```python
from build123d import *

# Parameters (mm, degrees)
SKETCH_W        = 110
SKETCH_H        = 25
PAD_DEPTH       = 70
POCKET_DEPTH    = 22.5
SKETCH002_W     = 20
SKETCH002_H     = 22.5
POCKET001_DEPTH = 70.001
SKETCH003_W     = 15
SKETCH003_H     = 15
SKETCH003_R     = 1.5
PAD001_DEPTH    = 2.5
SKETCH004_W     = 15
SKETCH004_H     = 15
SKETCH004_R     = 1.5
PAD002_DEPTH    = 2.5
POCKET002_DEPTH = 2.5
SKETCH006_W     = 26
SKETCH006_H     = 14.5
POCKET003_DEPTH = 2.5
SKETCH007_W     = 20
SKETCH007_H     = 2.5
PAD003_DEPTH    = 22.5
SKETCH008_W     = 20
SKETCH008_H     = 2.5
PAD004_DEPTH    = 22.5
SKETCH009_R     = 1.5
PAD005_DEPTH    = 0.15
SKETCH010_R     = 1.5
PAD006_DEPTH    = 0.15


with BuildPart() as part:
    # Sketch → Pad (new body)
    with BuildSketch(Plane.YZ):
        with Locations((55, 12.5)):
            Rectangle(SKETCH_W, SKETCH_H)
    extrude(amount=PAD_DEPTH)

    # Sketch001 (on Face3 of Pad) → Pocket (cut)
    with BuildSketch(Plane(origin=(0, 0, 25), x_dir=(0, -1, 0), z_dir=(0, 0, 1))):
        Polygon((-107.5, 2.5), (-2.5, 2.5), (-2.5, 67.5), (-107.5, 67.5), (-110, 67.5), (-110, 2.5), align=None)
    extrude(amount=-POCKET_DEPTH, mode=Mode.SUBTRACT)

    # Sketch002 (on Face5 of Pocket) → Pocket001 (cut, through all)
    with BuildSketch(Plane.YZ.offset(70)):
        with Locations((100, 13.75)):
            Rectangle(SKETCH002_W, SKETCH002_H)
    extrude(amount=-POCKET001_DEPTH, mode=Mode.SUBTRACT)

    # Sketch003 (on Face5 of Pocket001) → Pad001 (join, symmetric)
    with BuildSketch(Plane.YZ.offset(70)):
        with Locations((40, 27.5)):
            Rectangle(SKETCH003_W, SKETCH003_H)
        with Locations((40, 30)):
            Circle(SKETCH003_R, mode=Mode.SUBTRACT)
    extrude(amount=PAD001_DEPTH, both=True)

    # Sketch004 (on Face4 of Pad001) → Pad002 (join, symmetric)
    with BuildSketch(Plane(origin=(0, 0, 0), x_dir=(0, 1, 0), z_dir=(-1, 0, 0))):
        with Locations((40, -27.5)):
            Rectangle(SKETCH004_W, SKETCH004_H)
        with Locations((40, -30)):
            Circle(SKETCH004_R, mode=Mode.SUBTRACT)
    extrude(amount=PAD002_DEPTH, both=True)

    # Sketch005 → Pocket002 (cut)
    with BuildSketch(Plane.YX):
        with BuildLine():
            ThreePointArc((70, 47.5), (57.5, 35), (70, 22.5))
            Line((70, 22.5), (110, 22.5))
            ThreePointArc((110, 22.5), (122.5, 35), (110, 47.5))
            Line((70, 47.5), (110, 47.5))
        make_face()
    extrude(amount=-POCKET002_DEPTH, mode=Mode.SUBTRACT)

    # Sketch006 (on Face2 of Pocket002) → Pocket003 (cut)
    with BuildSketch(Plane(origin=(0, 0, 0), x_dir=(0, 1, 0), z_dir=(-1, 0, 0))):
        with Locations((77, -17.75)):
            Rectangle(SKETCH006_W, SKETCH006_H)
    extrude(amount=-POCKET003_DEPTH, mode=Mode.SUBTRACT)

    # Sketch007 (on Face17 of Pocket003) → Pad003 (join)
    with BuildSketch(Plane(origin=(0, 0, 2.5), x_dir=(0, -1, 0), z_dir=(0, 0, 1))):
        with Locations((-100, 1.25)):
            Rectangle(SKETCH007_W, SKETCH007_H)
    extrude(amount=PAD003_DEPTH)

    # Sketch008 (on Face15 of Pad003) → Pad004 (join)
    with BuildSketch(Plane(origin=(0, 0, 2.5), x_dir=(0, -1, 0), z_dir=(0, 0, 1))):
        with Locations((-100, 68.75)):
            Rectangle(SKETCH008_W, SKETCH008_H)
    extrude(amount=PAD004_DEPTH)

    # Sketch009 (on Face17 of Pad004) → Pad005 (join)
    with BuildSketch(Plane.YZ.offset(2.5)):
        Polygon((110, 25), (110, 2.5), (2.5, 2.5), (2.5, 25), (32.5, 25), (32.5, 35), (47.5, 35), (47.5, 25), (64, 25), (64, 10.5), (90, 10.5), (90, 25), align=None)
        with Locations((40, 30)):
            Circle(SKETCH009_R, mode=Mode.SUBTRACT)
    extrude(amount=PAD005_DEPTH)

    # Sketch010 (on Face11 of Pad005) → Pad006 (join)
    with BuildSketch(Plane(origin=(67.5, 0, 0), x_dir=(0, 1, 0), z_dir=(-1, 0, 0))):
        Polygon((2.5, -2.5), (110, -2.5), (110, -25), (47.5, -25), (47.5, -35), (32.5, -35), (32.5, -25), (2.5, -25), align=None)
        with Locations((40, -30)):
            Circle(SKETCH010_R, mode=Mode.SUBTRACT)
    extrude(amount=PAD006_DEPTH)


solid = part.part
```
Could you check a few things on this model? Use its own coordinates, in mm. A direction names the side the tool comes from. Round coordinates to 2 decimals unless told otherwise and drop trailing zeros. Write each loop counter-clockwise with the first axis right and the second up, starting at its lowest first coordinate (ties: lowest second). Pieces come first, ordered by that corner, then holes. Notation, with made-up numbers: M 22,14.25 L 41,14.25 A11 cw 41,29.25 Z; hole C 37,43 d3. An arc over 180 degrees is marked long. Write each question's results on one line, items separated by ' | '. Start each with the question number.
1. I need wall thicknesses on L1, parallel to Y at x = 0, z = 30; L2, parallel to X at y = 37, z = 11; L3, parallel to Z at x = 1.15, y = 40. Which ranges of each line are inside material? Lowest first, please. Write a range as from..to.
2. Thinking about a two-plate mould opening in Z: for faces 4 (the face through (69.96, 38.89, 28.99)), 5 (the face through (35, 54, 0)), 6 (the face through (1, 77, 10.5)), 7 (the face through (0, 32.5, 29)), which applies, +Z half, -Z half, draft (parallel to the pull), parting line (faces both ways), or undercut?
3. Imagine slicing it at D-D on y = 28.5. List the corners of the cut face in (x, z) for me, and give its area (3 significant figures).
4. Imagine slicing it at C-C on z = 30. List the corners of the cut face in (x, y) for me, and give its area (3 significant figures).
5. On a 3-axis mill with a long thin cutter (end or side, diameter ignored), from which of +Z, -Z, +X, -X, +Y, -Y can I reach the whole of each face in a straight line? I mean faces 1 (the face through (1, 56, 25)), 2 (the face through (1, 64, 18)), 3 (the face through (35, 55, 2.5)). Say none if no direction works.
6. Imagine slicing it at B-B on y = 40. List the corners of the cut face in (x, z) for me, and give its area (3 significant figures).
7. Imagine slicing it at A-A on z = 17. List the corners of the cut face in (x, y) for me, and give its area (3 significant figures).
8. I'm going to push flat-ended pins straight in: pin 1 Ø1.2 at (y, z) = (81, 2) entering from -X; pin 2 Ø1.5 at (x, z) = (-0.5, 28) entering from +Y; pin 3 Ø2 at (x, z) = (6.5, 4.5) entering from +Y. Where does each tip first touch, or does it pass through?
Result sheet:
1) L1: y = 32.5..38.5, 41.5..47.5 | L2: x = 0..2.65, 67.35..70 | L3: z = 0..28.5, 31.5..35
2) face 4: undercut | face 5: -Z half | face 6: +Z half | face 7: draft
3) outline: M 0,0 L 70,0 L 70,25 L 67.35,25 L 67.35,2.5 L 2.65,2.5 L 2.65,25 L 0,25 Z | area: 294 mm^2
4) outline: M -2.5,32.5 L 2.65,32.5 L 2.65,38.5 L -2.5,38.5 Z; M -2.5,41.5 L 2.65,41.5 L 2.65,47.5 L -2.5,47.5 Z; M 67.35,32.5 L 72.5,32.5 L 72.5,38.5 L 67.35,38.5 Z; M 67.35,41.5 L 72.5,41.5 L 72.5,47.5 L 67.35,47.5 Z | area: 124 mm^2
5) face 1: +Z, +X, -X, +Y | face 2: +Z, -X | face 3: +Z, +Y
6) outline: M -2.5,20 L 0,20 L 0,0 L 70,0 L 70,20 L 72.5,20 L 72.5,28.5 L 67.35,28.5 L 67.35,2.5 L 2.65,2.5 L 2.65,28.5 L -2.5,28.5 Z; M -2.5,31.5 L 2.65,31.5 L 2.65,35 L -2.5,35 Z; M 67.35,31.5 L 72.5,31.5 L 72.5,35 L 67.35,35 Z | area: 391 mm^2
7) outline: M 0,0 L 70,0 L 70,110 L 67.35,110 L 67.35,2.5 L 2.65,2.5 L 2.65,64 L 0,64 Z; M 0,90 L 2.65,90 L 2.65,110 L 0,110 Z | area: 676 mm^2
8) pin 1: stops at x = 0 | pin 2: stops at y = 47.5 | pin 3: stops at y = 2.5
